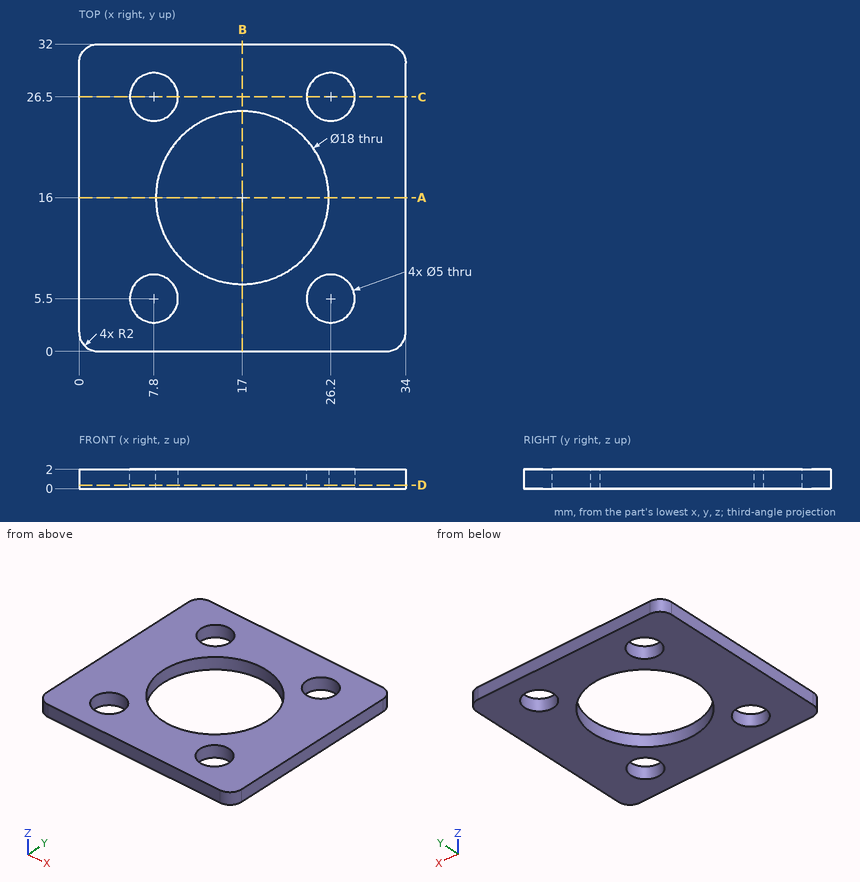
Study the drawing (mm; zero at the part's minimum x, y, z) and answer. Round coordinates to 2 decimals unless told otherwise and drop trailing zeros. Loops run counter-clockwise (first coordinate to the right, second up) from the corner with the lowest first, then second, coordinate; pieces in that order, holes last. Notation, with made-up numbers: (68.5, -35.5) - (78.5, -35.5) arc R11 ccw to (78.5, -21.5) - close; hole circle Ø2 at (-25, 82). An arc over 180 degrees is marked (long way). Use one line per item in the form item = value. Start each with the question number.
1. The part is cut by section C-C on y = 26.5. Determine the outline of the cut face in (x, z), then the cut area to 3 significant figures.
2. The part is cut by section D-D on z = 0.35. Determine the outline of the cut face in (x, y).
3. Consider line 1 (Y direction, x = 26.2, z = 0.55); line 2 (Y direction, x = 17, z = 0.5); line 3 (X direction, y = 10, z = 1.2). Determine where each line is inside the solid, lowest interval first. Write a range as [from, to].
4. The part is cut by section B-B on x = 17. Determine the outline of the cut face in (y, z).
5. The part is cut by section A-A on y = 16. Determine the outline of the cut face in (x, z), then the cut area to 3 significant figures.
Geometry check:
q1.outline = (0, 0) - (5.3, 0) - (5.3, 2) - (0, 2) - close; (10.3, 0) - (23.7, 0) - (23.7, 2) - (10.3, 2) - close; (28.7, 0) - (34, 0) - (34, 2) - (28.7, 2) - close
q1.area = 48.0 mm^2
q2.outline = (0, 2) arc R2 ccw to (2, 0) - (32, 0) arc R2 ccw to (34, 2) - (34, 30) arc R2 ccw to (32, 32) - (2, 32) arc R2 ccw to (0, 30) - close; hole circle Ø5 at (7.8, 5.5); hole circle Ø5 at (7.8, 26.5); hole circle Ø18 at (17, 16); hole circle Ø5 at (26.2, 5.5); hole circle Ø5 at (26.2, 26.5)
q3.line_1 = [0, 3], [8, 24], [29, 32]
q3.line_2 = [0, 7], [25, 32]
q3.line_3 = [0, 10.29], [23.71, 34]
q4.outline = (0, 0) - (7, 0) - (7, 2) - (0, 2) - close; (25, 0) - (32, 0) - (32, 2) - (25, 2) - close
q5.outline = (0, 0) - (8, 0) - (8, 2) - (0, 2) - close; (26, 0) - (34, 0) - (34, 2) - (26, 2) - close
q5.area = 32.0 mm^2
